```python
from build123d import *

# Parameters (mm, degrees)
BOSS_EXTRUDE1_DEPTH = 10
FILLET1_R           = 2
SKETCH2_W           = 26.5
SKETCH2_H           = 22
BOSS_EXTRUDE2_DEPTH = 15.88
SKETCH3_R           = 7.9375
BOSS_EXTRUDE3_DEPTH = 10


with BuildPart() as part:
    # Sketch1 → Boss-Extrude1 (new body)
    with BuildSketch(Plane(origin=(0, 0, 0), x_dir=(0, 0, -1), z_dir=(1, 0, 0))):
        Polygon((-26.5, -27.5), (-26.5, -5.5), (-23.5, -5.5), (-23.5, -15.5), (-20.5, -15.5), (-20.5, -12.5), (-17.5, -12.5), (-17.5, -17.5), (-12, -17.5), (-12, -20.5), (-15, -20.5), (-15, -23.5), (0, -23.5), (0, -27.5), align=None)
    extrude(amount=BOSS_EXTRUDE1_DEPTH)

    # Fillet1
    fillet1_edges = [part.edges().sort_by_distance(p)[0] for p in [
        (5, -12.5, 17.5),
        (5, -17.5, 12),
    ]]
    fillet(fillet1_edges, radius=FILLET1_R)

    # Sketch2 → Boss-Extrude2 (add)
    with BuildSketch(Plane.ZY):
        with Locations((13.25, -16.5)):
            Rectangle(SKETCH2_W, SKETCH2_H)
    extrude(amount=BOSS_EXTRUDE2_DEPTH)

    # Sketch3 → Boss-Extrude3 (add)
    with BuildSketch(Plane(origin=(0, 0, 0), x_dir=(-1, 0, 0), z_dir=(0, 0, -1))):
        with BuildLine():
            Line((-10.00567497, -40.433161955), (-10, -23.5))
            Line((-10, -23.5), (15.88, -23.5))
            Line((15.88, -23.5), (15.882323576, -40.433162744))
            ThreePointArc((15.882323576, -40.433162744), (2.938323909, -53.3815), (-10.00567497, -40.433161955))
        make_face()
        with Locations(Location((2.938324303, -40.4375, 0), (0, 0, 90))):
            Circle(SKETCH3_R, mode=Mode.SUBTRACT)
    extrude(amount=-BOSS_EXTRUDE3_DEPTH)

    # Mirror1: part across plane


with BuildPart() as part_1:
    add(part.part)
    add(part.part.mirror(Plane(origin=(10, -23.5, 0), x_dir=(1, 0, 0), z_dir=(0, 0, 1))))


solid = part_1.part
```
Here's how the part is built. I have some questions about the finished solid (model axes, mm). A direction names the side the tool comes from. Give positions to 0.01 mm unless a question says otherwise; leave off trailing zeros. Loops run counter-clockwise (first coordinate to the right, second up) from the corner with the lowest first, then second, coordinate; pieces in that order, holes last. Notation, with made-up numbers: M -25.5,-33 L -0.5,-33 A29 ccw -0.5,2 Z; hole C -7.5,67.25 d11. An arc over 180 degrees is marked long. Return JSON: item names as keys, results as strings.
Item 1: Imagine slicing it at B-B on x = -6.5. List the corners of the cut face in (y, z) for me.
A:
{"outline": "M -52.88,-10 L -47.53,-10 L -47.53,10 L -52.88,10 Z; M -33.34,-10 L -27.5,-10 L -27.5,-26.5 L -5.5,-26.5 L -5.5,26.5 L -27.5,26.5 L -27.5,10 L -33.34,10 Z"}
Item 2: On a 3-axis mill with a long thin cutter (end or side, diameter ignored), from which of +Z, -Z, +X, -X, +Y, -Y can I reach the whole of each face in a straight line? I mean faces 1 (the flat face through (5, -20.5, -13)), 2 (the flat face through (5, -15.5, -22)), 3 (the cylindrical face through (-5.978, -33.105, 0.14)), 4 (the flat face through (-9, -35, 10)). Say none if no direction works.
A:
{"face 1": "+X", "face 2": "+X, +Y", "face 3": "+Z, -Z", "face 4": "+Z, +X, -X, -Y"}
Item 3: Imagine slicing it at C-C on z = 7. List the corners of the cut face in (x, y) for me (1 decimal).
A:
{"outline": "M -15.9,-40.4 A12.9 ccw 10,-40.4 L 10,-23.5 L 0,-23.5 L 0,-5.5 L -15.9,-5.5 L -15.9,-23.5 Z; hole C -2.9,-40.4 d15.9"}
Item 4: I'm going to push flat-ended pins straight in: pin 1 Ø5 at (x, z) = (-4, -15) entering from -Y; pin 2 Ø4 at (y, z) = (-29.5, 8) entering from +X; pin 3 Ø4 at (x, z) = (-9.5, 4.5) entering from -Y. Where does each tip first touch, or does it pass through?
A:
{"pin 1": "stops at y = -27.5", "pin 2": "stops at x = 10", "pin 3": "stops at y = -52.55"}
Item 5: Imagine slicing it at D-D on y = -10. List the corners of the cut face in (x, z) for me, then the cut area to 3 significant figures.
A:
{"outline": "M -15.88,-26.5 L 10,-26.5 L 10,-23.5 L 0,-23.5 L 0,23.5 L 10,23.5 L 10,26.5 L -15.88,26.5 Z", "area": "902 mm^2"}
Item 6: Thinking about a two-plate mould opening in Y: for faces 5 (the flat face through (5, -22, 15)), 6 (the flat face through (-3, -27.5, 18)), 7 (the flat face through (5, -10, -23.5)), 8 (the cylindrical face through (5.07, -13.07, 18.1)), which applies, released by +Y, released by -Y, zero draft, split by the parting line, or undercut?
A:
{"face 5": "undercut", "face 6": "released by -Y", "face 7": "zero draft", "face 8": "released by +Y"}
Item 7: Imagine slicing it at A-A on y = -33.5. List the corners of the cut face in (x, z) for me.
A:
{"outline": "M -15.88,-10 L -6.8,-10 L -6.8,10 L -15.88,10 Z; M 0.92,-10 L 10,-10 L 10,10 L 0.92,10 Z"}
Item 8: Please list where these lines run through material, in increasing order: line 1 (Z direction, x = 0.75, y = -22.5); line 2 (Z direction, x = 5.5, y = -20); line 3 (Y direction, x = -1, z = 19).
A:
{"line 1": "z = -26.5 to -15, 15 to 26.5", "line 2": "z = -26.5 to -12, 12 to 26.5", "line 3": "y = -27.5 to -5.5"}
